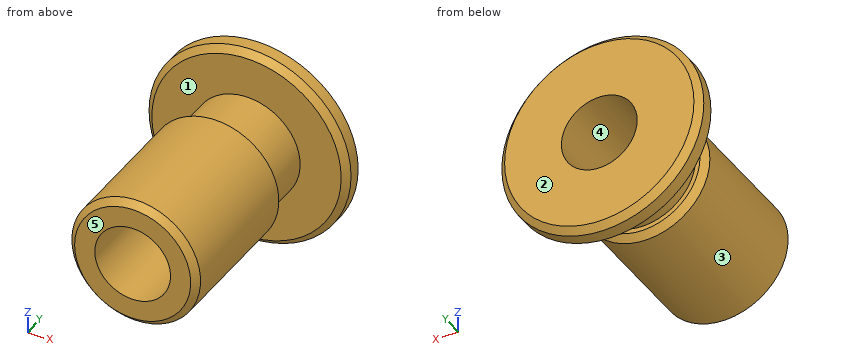
from build123d import *

# Parameters (mm, degrees)
F2_SIZE = 0.5


with BuildPart() as f1:
    # F0 (on Top) → F1 (revolve)
    with BuildSketch(Plane.XY):
        Polygon((-5.1, 12), (-5.1, 0), (-3, 0), (-3, 18), (-8, 18), (-8, 16), (-4.25, 16), (-4.25, 12), align=None)
    revolve(axis=Axis((0, 9, 0), (0, 1, 0)))

    # F2
    f2_edges = [f1.edges().sort_by_distance(p)[0] for p in [
        (8, 18, 0),
        (8, 16, 0),
        (-8, 17, 0),
        (5.1, 12, 0),
        (5.1, 0, 0),
        (-5.1, 6, 0),
    ]]
    chamfer(f2_edges, length=F2_SIZE)


solid = f1.part
Read the model definition and answer for the solid it produces. Units are mm, in the model's axes. Face numbers are marked on the shaded views. A direction names the side the tool comes from. Give positions to 0.01 mm unless a question says otherwise; leave off trailing zeros. Loops run counter-clockwise (first coordinate to the right, second up) from the corner with the lowest first, then second, coordinate; pieces in that order, holes last. Notation, with made-up numbers: (46, 65) - (60, 65) arc R25 ccw to (60, 86) - close; hole circle Ø11 at (28, -1.5). An arc over 180 degrees is marked (long way). Answer as CSV lines item,"result". Start each with the question number.
1) Find section B-B (z = 0). Write down the section's boundary in (x, y), then the cut area to 3 significant figures.
2) Find section D-D (y = 9). Write down the section's boundary in (x, z), then the cut area to 3 significant figures.
3) Determine the mould class of the marked faces 3, 4 and 5 for opening direction Z: released by +Z, released by -Z, zero draft, split by the parting line, or undercut.
4) Find section A-A (x = 0). Write down the section's boundary in (y, z), then the cut area to 3 significant figures.
5) Find section C-C (y = 13.25). Write down the section's boundary in (x, z), then the cut area to 3 significant figures.
6) Each of these flat-tipped pins is pushed along its axis until it touches: pin 1 Ø5 at (y, z) = (2.5, 5.5) entering from +X; pin 2 Ø5 at (y, z) = (15, -2.5) entering from +X; pin 3 Ø5 at (x, y) = (0, 4) entering from +Z. Where does it stop, or does it pass through?
7) Which of the six approach directions +Z, -Z, +X, -X, +Y, -Y give full straight-line access (tool end or side, diameter ignored) to the marked faces 1 and 2?
8) Straight lines are drawn through the part: L1, parallel to Z at x = 0, y = 10.75; L2, parallel to Y at x = -3.75, z = 5.5; L3, parallel to Y at x = 0.75, z = 5. For each, find the intervals that lie inside material, in ascending order. Write a range as from..to.
Findings below:
1,outline,"(-8, 16.5) - (-7.5, 16) - (-4.25, 16) - (-4.25, 12) - (-4.6, 12) - (-5.1, 11.5) - (-5.1, 0.5) - (-4.6, 0) - (-3, 0) - (-3, 18) - (-7.5, 18) - (-8, 17.5) - close; (3, 0) - (4.6, 0) - (5.1, 0.5) - (5.1, 11.5) - (4.6, 12) - (4.25, 12) - (4.25, 16) - (7.5, 16) - (8, 16.5) - (8, 17.5) - (7.5, 18) - (3, 18) - close"
1,area,"79.4 mm^2"
2,outline,"circle Ø10.2 at (0, 0); hole circle Ø6 at (0, 0)"
2,area,"53.4 mm^2"
3,face 3,"split by the parting line"
3,face 4,"undercut"
3,face 5,"zero draft"
4,outline,"(0, -4.6) - (0.5, -5.1) - (11.5, -5.1) - (12, -4.6) - (12, -4.25) - (16, -4.25) - (16, -7.5) - (16.5, -8) - (17.5, -8) - (18, -7.5) - (18, -3) - (0, -3) - close; (0, 3) - (18, 3) - (18, 7.5) - (17.5, 8) - (16.5, 8) - (16, 7.5) - (16, 4.25) - (12, 4.25) - (12, 4.6) - (11.5, 5.1) - (0.5, 5.1) - (0, 4.6) - close"
4,area,"79.4 mm^2"
5,outline,"circle Ø8.5 at (0, 0); hole circle Ø6 at (0, 0)"
5,area,"28.5 mm^2"
6,pin 1,"x = 4.12"
6,pin 2,"x = 7.98"
6,pin 3,"z = 5.1"
7,face 1,"none"
7,face 2,"+Z, -Z, +X, -X, +Y"
8,L1,"-5.1..-3, 3..5.1"
8,L2,"16..18"
8,L3,"0.46..11.54, 16..18"
